Geometry check sheet. Reference: the model listing, model coordinates, mm. A direction names the side the tool comes from. Round coordinates to 2 decimals unless told otherwise and drop trailing zeros. Order: outer loops, then holes, each group sorted by start corner. A loop starts at its lowest first (then second) coordinate and runs counter-clockwise, first axis right, second up. Notation, with made-up numbers: (7.5, 48) - (54.5, 48) arc R25 cw to (54.5, 75) - close; hole circle Ø9 at (21, 62.25). An arc over 180 degrees is marked (long way). Return JSON: item names as keys, results as strings. Group by question number.
Q1. Draft check along X on faces 3 (the flat face through (4, 0, 4)), 4 (the cylindrical face through (-1.5, 0.07, 6.03)), 5 (the cylindrical face through (-3, -8, 4)), 6 (the flat face through (2, 0, 8)). Enter one of: pulls with the +X half, pulls with the -X half, needs draft (parallel to the pull), parting line crosses it, or undercut.
Q2. Sectioned sample at D-D, the plane x = 1.25. Record the cut outline in (y, z), then the cut area to 3 significant figures.
Q3. Sectioned sample at B-B, the plane y = 0. Record the cut outline in (x, z).
Q4. Tool access check on faces 1 (the cylindrical face through (0, -2, 2)), 2 (the cylindrical face through (3, 8, 4)). Record the directions out of +Z, -Z, +X, -X, +Y, -Y that give a thin tool (end or side, any length) a straight path to the whole face; none if there is none.
Q5. Gauge pin test, flat ends, axial feed: pin 1 Ø1.8 at (x, y) = (0, 0) entering from +Z; pin 2 Ø4 at (x, z) = (2.5, 3.5) entering from +Y. Record the tip position at first contact, or that the pin passes through.
Q6. Material ranges on line 1 along Y through (x, z) = (0, 2.15); line 2 along X through (y, z) = (0.75, 7.25); line 3 along Z through (x, y) = (0, -0.75), recorded low to high.
Q7. Sectioned sample at A-A, the plane z = 1.25. Record the cut outline in (x, y), then the cut area to 3 significant figures.
Q8. Sectioned sample at C-C, the plane z = 6.5. Record the cut outline in (x, y).
```python
from build123d import *

# Parameters (mm, degrees)
F0_W        = 8
F0_H        = 20
F1_DEPTH    = 8
F2_T1_DEPTH = 33
F3_R        = 1.5
F4_DEPTH    = 7
F5_R        = 2
F5_R_2      = 1.5
F6_DEPTH    = 3


# Not quite as in the source:
# - a fillet or chamfer that OpenCascade refuses, or shapes differently, is made with other operations: its cross-section is extruded or revolved along the edge and cut away or added


with BuildPart() as f1:
    # F0 (on Top) → F1 (new body)
    with BuildSketch(Plane.XY):
        Rectangle(F0_W, F0_H)
    extrude(amount=F1_DEPTH)

    # F2: fillet of radius 5 on 4 edges, made by hand

    # F2_s2 → F2_t1 (cut)
    with BuildSketch(Plane.XY.offset(-12.5)):
        with BuildLine():
            ThreePointArc((4, -5), (2.5355339059, -8.5355339059), (-1, -10))
            Line((-1, -10), (4, -10))
            Line((4, -10), (4, -5))
        make_face()
        with BuildLine():
            ThreePointArc((-4, -5), (-2.5355339059, -8.5355339059), (1, -10))
            Line((1, -10), (-4, -10))
            Line((-4, -10), (-4, -5))
        make_face()
        with BuildLine():
            ThreePointArc((4, 5), (2.5355339059, 8.5355339059), (-1, 10))
            Line((-1, 10), (4, 10))
            Line((4, 10), (4, 5))
        make_face()
        with BuildLine():
            ThreePointArc((1, 10), (-2.5355339059, 8.5355339059), (-4, 5))
            Line((-4, 5), (-4, 10))
            Line((-4, 10), (1, 10))
        make_face()
    extrude(amount=F2_T1_DEPTH, mode=Mode.SUBTRACT)

    # F3 (on face) → F4 (cut)
    with BuildSketch(Plane.XY.offset(8)):
        Circle(F3_R)
    extrude(amount=-F4_DEPTH, mode=Mode.SUBTRACT)

    # F5 (on face) → F6 (cut)
    with BuildSketch(Plane.XY.offset(1)):
        Circle(F5_R)
        Circle(F5_R_2, mode=Mode.SUBTRACT)
    extrude(amount=F6_DEPTH, mode=Mode.SUBTRACT)


solid = f1.part
```
Reply:
{
 "1": {"face 3": "pulls with the +X half", "face 4": "undercut", "face 5": "pulls with the -X half", "face 6": "needs draft"},
 "2": {"outline": "(-9.47, 0) - (9.47, 0) - (9.47, 8) - (0.83, 8) - (0.83, 4) - (1.56, 4) - (1.56, 1) - (-1.56, 1) - (-1.56, 4) - (-0.83, 4) - (-0.83, 8) - (-9.47, 8) - close", "area": "135 mm^2"},
 "3": {"outline": "(-4, 0) - (4, 0) - (4, 8) - (1.5, 8) - (1.5, 4) - (2, 4) - (2, 1) - (-2, 1) - (-2, 4) - (-1.5, 4) - (-1.5, 8) - (-4, 8) - close"},
 "4": {"face 1": "none", "face 2": "+Z, -Z, +X, +Y"},
 "5": {"pin 1": "z = 1", "pin 2": "y = 9.77"},
 "6": {"line 1": "-9.9 to -2, 2 to 9.9", "line 2": "-4 to -1.3, 1.3 to 4", "line 3": "0 to 1"},
 "7": {"outline": "(-4, -5) arc R5 ccw to (0, -9.9) arc R5 ccw to (4, -5) - (4, 5) arc R5 ccw to (0, 9.9) arc R5 ccw to (-4, 5) - close; hole circle Ø4 at (0, 0)", "area": "126 mm^2"},
 "8": {"outline": "(-4, -5) arc R5 ccw to (0, -9.9) arc R5 ccw to (4, -5) - (4, 5) arc R5 ccw to (0, 9.9) arc R5 ccw to (-4, 5) - close; hole circle Ø3 at (0, 0)"}
}
